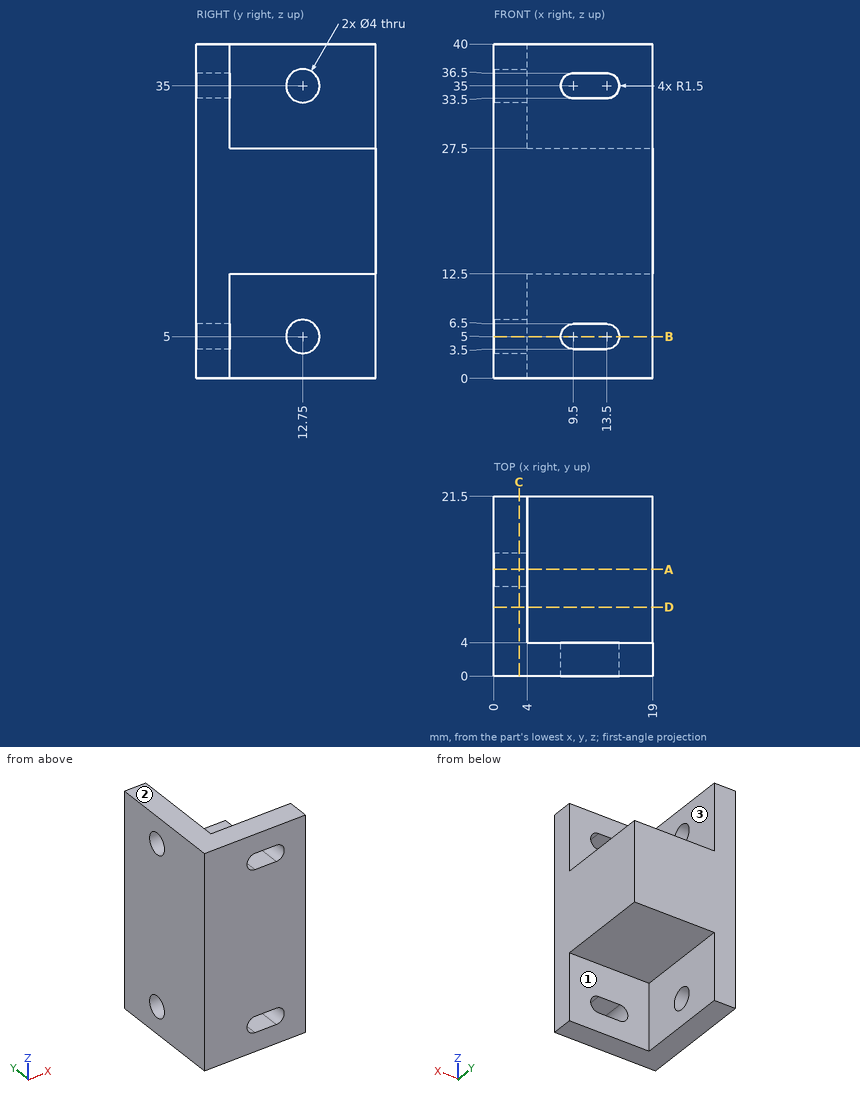
Check sheet for the drawn part. Datum: minimum x, y, z corner. Units: mm. A direction names the side the tool comes from. Give positions to 0.01 mm unless a question says otherwise; leave off trailing zeros. Write each loop counter-clockwise with the first axis right and the second up, starting at its lowest first coordinate (ties: lowest second). Pieces come first, ordered by that corner, then holes.
(1) Cross-section at A-A (y = 12.75). Enter the section's corners in (x, z), plus the area to 3 significant figures.
(2) Gauge pin test, flat ends, axial feed: pin 1 (1 mm diameter, centred on x = 16.5, z = 33.5, fed in from -Y); pin 2 (6 mm diameter, centred on y = 15, z = 9, fed in from +X); pin 3 (1.5 mm diameter, centred on x = 14.5, y = 14.5, fed in from -Z); pin 4 (10 mm diameter, centred on x = 10, z = 33, fed in from +Y). Record the tip position at first contact, or that the pin passes through.
(3) Access from +Z, -Z, +X, -X, +Y, -Y to the whole of each face (thin tool, end or side, straight path). Record for the marked faces 1, 2 and 3.
(4) Cross-section at B-B (z = 5). Enter the section's corners in (x, y).
(5) Cross-section at D-D (y = 8.25). Enter the section's corners in (x, z).
(6) Cross-section at C-C (x = 3). Enter the section's corners in (y, z).
(7) Material ranges on line 1 (Z direction, x = 12.75, y = 3.25); line 2 (Y direction, x = 0.85, z = 35); line 3 (Y direction, x = 17.75, z = 8), recorded low to high.
Worked out:
1. outline: (0, 0) - (4, 0) - (4, 3) - (0, 3) - close; (0, 7) - (4, 7) - (4, 12.5) - (19, 12.5) - (19, 27.5) - (4, 27.5) - (4, 33) - (0, 33) - close; (0, 37) - (4, 37) - (4, 40) - (0, 40) - close
1. area: 353 mm2
2. pin 1: stops at y = 0
2. pin 2: stops at x = 4
2. pin 3: stops at z = 12.5
2. pin 4: stops at y = 4
3. face 1: -Z, +X, +Y
3. face 2: +Z, +X, -X, +Y, -Y
3. face 3: +Z, +X, +Y
4. outline: (0, 0) - (8, 0) - (8, 4) - (4, 4) - (4, 10.75) - (0, 10.75) - close; (0, 14.75) - (4, 14.75) - (4, 21.5) - (0, 21.5) - close; (15, 0) - (19, 0) - (19, 4) - (15, 4) - close
5. outline: (0, 0) - (4, 0) - (4, 12.5) - (19, 12.5) - (19, 27.5) - (4, 27.5) - (4, 40) - (0, 40) - close
6. outline: (0, 0) - (21.5, 0) - (21.5, 40) - (0, 40) - close; hole circle Ø4 at (12.75, 5); hole circle Ø4 at (12.75, 35)
7. line 1: z = 0 to 3.5, 6.5 to 33.5, 36.5 to 40
7. line 2: y = 0 to 10.75, 14.75 to 21.5
7. line 3: y = 0 to 4
